```python
from build123d import *

# Parameters (mm, degrees)
F1_DEPTH = 0.508
F3_SIZE2 = 1.778
F3_SIZE  = 0.2286
F4_DEPTH = 25.4


with BuildPart() as f1:
    # F0 (on Top) → F1 (new body)
    with BuildSketch(Plane.XY):
        Polygon((20.530576, 0), (0, 0), (5.279291, -9.144), (25.809866, -9.144), align=None)
    extrude(amount=F1_DEPTH)

    # F3
    f3_edges = [f1.edges().sort_by_distance(p)[0] for p in [
        (15.544579, -9.144, 0.508),
        (15.544579, -9.144, 0),
    ]]
    chamfer(f3_edges, length=F3_SIZE, length2=F3_SIZE2)

    # F2 (on face) → F4 (cut)
    with BuildSketch(Plane.XY.offset(0.508)):
        Polygon((25.301866, -9.144), (25.809866, -9.144), (24.636691, -7.112), align=None)
    extrude(amount=-F4_DEPTH, mode=Mode.SUBTRACT)


solid = f1.part
```
The model under review builds one solid part; all positions refer to its coordinate system, in mm. Give positions to 0.01 mm unless a question says otherwise; leave off trailing zeros. Write each loop counter-clockwise with the first axis right and the second up, starting at its lowest first coordinate (ties: lowest second). Pieces come first, ordered by that corner, then holes.
(1) For P1, Ø2, axis at x = 22, y = -1, coming from the -Z side, flat-tipped, find the tip position at first contact; note if it passes through.
(2) Consider section D-D, the plane x = 2.5. Give the boundary of the cut face in (y, z), and give its area (3 significant figures).
(3) To check wall thickness, follow L1, parallel to X at y = -0.75, z = 0.1; L2, parallel to X at y = -2.5, z = 0.15; L3, parallel to Y at x = 3.75, z = 0.3. State the ranges of each line that lie inside material, in increasing order.
(4) Consider section B-B, the plane z = 0.1. Give the boundary of the cut face in (x, y).
(5) Consider section A-A, the plane x = 8.25. Give the boundary of the cut face in (y, z), and give its area (3 significant figures).
(6) Consider section C-C, the plane y = -5.75. Give the boundary of the cut face in (x, z).
Returned:
1. P1: stops at z = 0
2. outline: (-4.33, 0) - (0, 0) - (0, 0.51) - (-4.33, 0.51) - close
2. area: 2.20 mm2
3. L1: x = 0.43 to 20.96
3. L2: x = 1.44 to 21.97
3. L3: y = -6.5 to 0
4. outline: (0, 0) - (4.7, -8.14) - (24.97, -8.14) - (24.64, -7.11) - (20.53, 0) - close
5. outline: (-9.14, 0.23) - (-7.37, 0) - (0, 0) - (0, 0.51) - (-7.37, 0.51) - (-9.14, 0.28) - close
5. area: 4.24 mm2
6. outline: (3.32, 0) - (23.85, 0) - (23.85, 0.51) - (3.32, 0.51) - close
